Here's the drawing with two shaded views (mm, measured from the low corner). I have some questions. A direction names the side the tool comes from. Give positions to 0.01 mm unless a question says otherwise; leave off trailing zeros. Loops run counter-clockwise (first coordinate to the right, second up) from the corner with the lowest first, then second, coordinate; pieces in that order, holes last. Notation, with made-up numbers: (14, 19.25) - (58, 19.25) arc R13 ccw to (58, 35.25) - close; hole circle Ø10 at (28, -38). An arc over 180 degrees is marked (long way). Answer as a JSON object with one key per item and string values. Group by question number.
Item 1: Suppose I cut it at B-B on x = 29. Write out the boundary of the cut face in (y, z) (3 decimals), and give its area (3 significant figures).
Item 2: Please list where these lines run through material, in increasing order: L1, parallel to Z at x = 29, y = 2; L2, parallel to X at y = 50.85, z = 25.4; L3, parallel to Y at x = 22, z = 266 (3 decimals).
Item 3: Suppose I cut it at A-A on z = 25.4. Write out the boundary of the cut face in (x, y) (3 decimals), and give its area (3 significant figures).
Item 4: Which directions (+Z, -Z, +X, -X, +Y, -Y) give clear straight access to the entire face, cutting with the end or side of a thin tool? Please do the marked faces 4 and 5.
Item 5: Suppose I cut it at C-C on x = 16. Write out the boundary of the cut face in (y, z) (3 decimals), and give its area (3 significant figures).
Item 6: Will these pins go through, and if not, where does the flat tip stop? pin 1 (8 mm diameter, centred on x = 29, z = 324.6, fed in from +Y); pin 2 (14 mm diameter, centred on y = 36.5, z = 111.5, fed in from +X) (3 decimals); pin 3 (1 mm diameter, centred on x = 2.5, y = 14.5, fed in from -Z).
Item 7: Suppose I cut it at D-D on z = 79. Write out the boundary of the cut face in (x, y) (3 decimals).
Item 8: Thinking about a two-plate mould opening in Y: for the marked faces 1, 2 and 3, which applies, pulls with the +Y half, pulls with the -Y half, needs draft (parallel to the pull), parting line crosses it, or undercut?
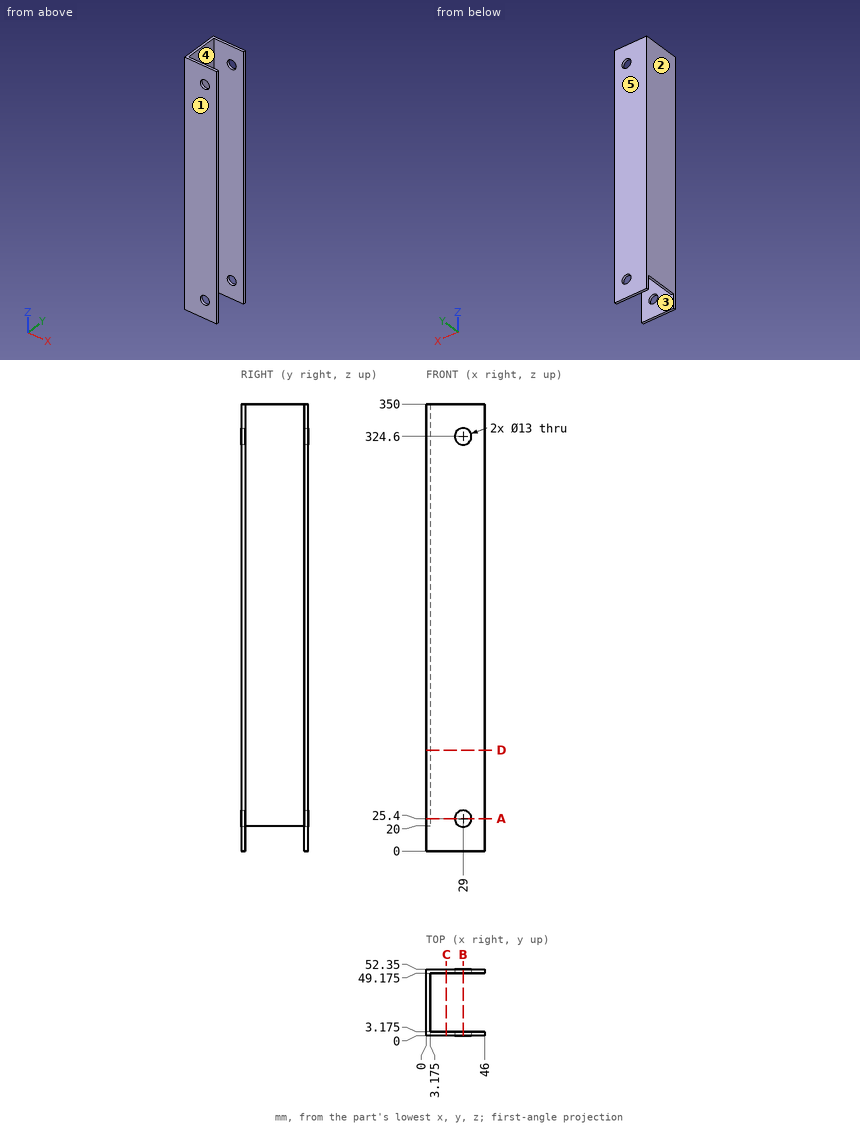
Worked out:
{
 "1": {"outline": "(0, 0) - (3.175, 0) - (3.175, 18.9) - (0, 18.9) - close; (0, 31.9) - (3.175, 31.9) - (3.175, 318.1) - (0, 318.1) - close; (0, 331.1) - (3.175, 331.1) - (3.175, 350) - (0, 350) - close; (49.175, 0) - (52.35, 0) - (52.35, 18.9) - (49.175, 18.9) - close; (49.175, 31.9) - (52.35, 31.9) - (52.35, 318.1) - (49.175, 318.1) - close; (49.175, 331.1) - (52.35, 331.1) - (52.35, 350) - (49.175, 350) - close", "area": "2,060 mm2"},
 "2": {"L1": "z = 0 to 18.9, 31.9 to 318.1, 331.1 to 350", "L2": "x = 0 to 22.5, 35.5 to 46", "L3": "y = 0 to 3.175, 49.175 to 52.35"},
 "3": {"outline": "(0, 0) - (22.5, 0) - (22.5, 3.175) - (3.175, 3.175) - (3.175, 49.175) - (22.5, 49.175) - (22.5, 52.35) - (0, 52.35) - close; (35.5, 0) - (46, 0) - (46, 3.175) - (35.5, 3.175) - close; (35.5, 49.175) - (46, 49.175) - (46, 52.35) - (35.5, 52.35) - close", "area": "356 mm2"},
 "4": {"face 4": "+Z, -Z, +X", "face 5": "+Z, -Z, +X, -X, +Y"},
 "5": {"outline": "(0, 0) - (3.175, 0) - (3.175, 350) - (0, 350) - close; (49.175, 0) - (52.35, 0) - (52.35, 350) - (49.175, 350) - close", "area": "2,220 mm2"},
 "6": {"pin 1": "passes through", "pin 2": "stops at x = 3.175", "pin 3": "stops at z = 20"},
 "7": {"outline": "(0, 0) - (46, 0) - (46, 3.175) - (3.175, 3.175) - (3.175, 49.175) - (46, 49.175) - (46, 52.35) - (0, 52.35) - close"},
 "8": {"face 1": "pulls with the -Y half", "face 2": "needs draft", "face 3": "undercut"}
}
